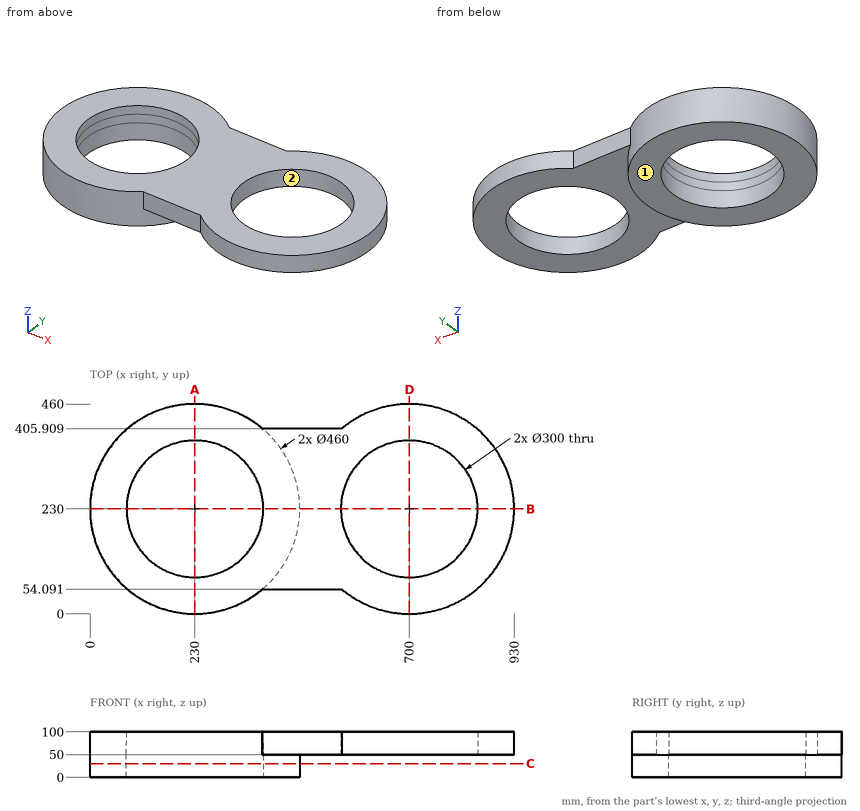
Geometry check sheet. Reference: drawing and pictorial views, mm from the part's lowest x, y, z. Give positions to 0.01 mm unless a question says otherwise; leave off trailing zeros. Order: outer loops, then holes, each group sorted by start corner. A loop starts at its lowest first (then second) coordinate and runs counter-clockwise, first axis right, second up. Notation, with made-up numbers: M 76.5,-2 L 112.5,-2 A13 cw 112.5,23 Z; hole C -30,75 d3. An arc over 180 degrees is marked long. Answer in a Markdown table with one row per item. Add a question column.
Q1. Thickness scan on L1, parallel to Y at x = 230, z = 69.5; L2, parallel to Y at x = 241, z = 75; L3, parallel to Z at x = 465, y = 151.5. Record the ranges inside material, lowest first.
Q2. Gauge pin test, flat ends, axial feed: pin 1 Ø10 at (x, z) = (501.5, 89) entering from -Y; pin 2 Ø3 at (y, z) = (135.5, 58.5) entering from +X; pin 3 Ø8 at (x, z) = (163, 74.5) entering from -Y. Record the tip position at first contact, or that the pin passes through.
Q3. Sectioned sample at A-A, the plane x = 230. Record the boundary of the cut face in (y, z), and give its area (3 significant figures).
Q4. Sectioned sample at B-B, the plane y = 230. Record the boundary of the cut face in (x, z), and give its area (3 significant figures).
Q5. Sectioned sample at C-C, the plane z = 30. Record the boundary of the cut face in (x, y).
Q6. Release check for a two-part mould opening along X. For the marked faces 1 and 2 record: released by +X, released by -X, zero draft, split by the parting line, or undercut.
Q7. Sectioned sample at D-D, the plane x = 700. Record the boundary of the cut face in (y, z).
Verdict:
| question | item | result |
|---|---|---|
| 1 | L1 | 0 to 80, 380 to 460 |
| 1 | L2 | 0.26 to 80.4, 379.6 to 459.74 |
| 1 | L3 | 50 to 100 |
| 2 | pin 1 | y = 54.09 |
| 2 | pin 2 | x = 910.36 |
| 2 | pin 3 | y = 8.8 |
| 3 | outline | M 0,0 L 80,0 L 80,100 L 0,100 Z; M 380,0 L 460,0 L 460,100 L 380,100 Z |
| 3 | area | 16,000 mm² |
| 4 | outline | M 0,0 L 80,0 L 80,100 L 0,100 Z; M 380,0 L 460,0 L 460,50 L 550,50 L 550,100 L 380,100 Z; M 850,50 L 930,50 L 930,100 L 850,100 Z |
| 4 | area | 24,500 mm² |
| 5 | outline | C 230,230 d460; hole C 230,230 d300 |
| 6 | face 1 | zero draft |
| 6 | face 2 | undercut |
| 7 | outline | M 0,50 L 80,50 L 80,100 L 0,100 Z; M 380,50 L 460,50 L 460,100 L 380,100 Z |
